from build123d import *

# Parameters (mm, degrees)
F0_W     = 10.859374
F0_H     = 12.747962
F1_DEPTH = 6.35


with BuildPart() as f1:
    # F0 (on Front) → F1 (new body)
    with BuildSketch(Plane.XZ):
        with Locations((-49.811488, 46.506466)):
            Rectangle(F0_W, F0_H)
        with BuildLine():
            ThreePointArc((-22.663044, 52.880447), (-33.522422, 50.119041), (-44.381801, 52.880447))
            Line((-44.381801, 52.880447), (-44.381801, 40.132485))
            ThreePointArc((-44.381801, 40.132485), (-33.58522, 42.779586), (-22.788638, 40.132485))
            Line((-22.788638, 40.132485), (-22.663044, 52.880447))
        make_face()
        Polygon((-12.275815, 52.880447), (-22.663044, 52.880447), (-22.788638, 40.132485), (-12.31831, 39.847307), align=None)
        Polygon((-12.31831, 39.847307), (-22.788638, 40.132485), (-22.788638, -13.626155), (-12.31831, -13.626155), align=None)
        with BuildLine():
            ThreePointArc((31.161692, 25.968079), (13.273611, 45.607102), (-12.275815, 52.880447))
            Line((-12.275815, 52.880447), (-12.31831, 39.847307))
            ThreePointArc((-12.31831, 39.847307), (10.459966, 36.160339), (31.161692, 25.968079))
        make_face()
        with BuildLine():
            Line((-12.31831, -13.626155), (-22.788638, -13.626155))
            ThreePointArc((-22.788638, -13.626155), (-27.217846, -15.308543), (-29.413201, -19.5072))
            Line((-29.413201, -19.5072), (-29.413201, -69.189601))
            ThreePointArc((-29.413201, -69.189601), (-28.519701, -72.668194), (-26.060402, -75.285599))
            Line((-26.060402, -75.285599), (-10.666025, -75.377978))
            ThreePointArc((-10.666025, -75.377978), (-8.094471, -72.573766), (-7.162803, -68.884797))
            Line((-7.162803, -68.884797), (-7.162803, -18.592801))
            ThreePointArc((-7.162803, -18.592801), (-8.738966, -15.069801), (-12.31831, -13.626155))
        make_face()
    extrude(amount=F1_DEPTH)


solid = f1.part
Geometry: final body of the model. Coordinates: model frame, mm. A direction names the side the tool comes from. Give positions to 0.01 mm unless a question says otherwise; leave off trailing zeros. Write each loop counter-clockwise with the first axis right and the second up, starting at its lowest first coordinate (ties: lowest second). Pieces come first, ordered by that corner, then holes. Notation, with made-up numbers: (4, 62.25) -> (46, 62.25) arc R26 ccw to (46, 94.25) -> close; hole circle Ø2 at (34.5, 36.5). An arc over 180 degrees is marked (long way). Answer in a Markdown table with one row per item.
(1) Ray query, line 1 along X through (y, z) = (-4.75, -57.5); line 2 along Z through (x, y) = (-48.5, -5); line 3 along X through (y, z) = (-4.25, -0.5). Return the intervals inside material, ascending. Write a range as [from, to].
Answers below:
| item | result |
|---|---|
| line 1 | [-29.41, -7.16] |
| line 2 | [40.13, 52.88] |
| line 3 | [-22.79, -12.32] |
(2) Section query B-B on y = -2.75. Return loops of the section in (x, z).
Answers below:
| item | result |
|---|---|
| outline | (-55.24, 40.13) -> (-44.38, 40.13) arc R23.34 cw to (-22.79, 40.13) -> (-22.79, -13.63) arc R6.67 ccw to (-29.41, -19.51) -> (-29.41, -69.19) arc R7.22 ccw to (-26.06, -75.29) -> (-10.67, -75.38) arc R7.77 ccw to (-7.16, -68.88) -> (-7.16, -18.59) arc R5.16 ccw to (-12.32, -13.63) -> (-12.32, 39.85) arc R77.97 cw to (31.16, 25.97) arc R48.51 ccw to (-12.28, 52.88) -> (-22.66, 52.88) arc R22.73 cw to (-44.38, 52.88) -> (-55.24, 52.88) -> close |
(3) Pin query (flat end, axial travel): pin 1 (1.9 mm diameter, centred on x = -48, y = -2.5, fed in from -Z); pin 2 (1.9 mm diameter, centred on y = -3.5, z = -33, fed in from +X); pin 3 (3 mm diameter, centred on x = 1.5, y = -5, fed in from +Z). Return the tip coordinate at first contact, or that it passes through.
Answers below:
| item | result |
|---|---|
| pin 1 | z = 40.13 |
| pin 2 | x = -7.16 |
| pin 3 | z = 51.3 |
(4) Set-up query: faces 1 (the flat face through (-50, -3, 40.132)), 2 (the flat face through (-7.163, -3, -44)), 3 (the flat face through (-12.318, -3, 13)), 4 (the cylindrical face through (-27.167, -3.131, -15.264)), 5 (the flat face through (-19, -6.35, -6)). Return all of +Z, -Z, +X, -X, +Y, -Y with unobstructed straight access to the full face (end or side cutting, diameter ignored); none if empty.
Answers below:
| item | result |
|---|---|
| face 1 | -Z, -X, +Y, -Y |
| face 2 | -Z, +X, +Y, -Y |
| face 3 | +Y, -Y |
| face 4 | -X, +Y, -Y |
| face 5 | +Z, -Z, +X, -X, -Y |
(5) Section query A-A on z = 36. Return loops of the section in (x, y), then the cut area to 3 significant figures.
Answers below:
| item | result |
|---|---|
| outline | (-22.79, -6.35) -> (-12.32, -6.35) -> (-12.32, 0) -> (-22.79, 0) -> close; (10.96, -6.35) -> (24.5, -6.35) -> (24.5, 0) -> (10.96, 0) -> close |
| area | 153 mm^2 |
(6) Draft query along Z for faces 6 (the flat face through (-55.241, -3, 46)), 7 (the flat face through (-22.789, -3, 14)), 8 (the cylindrical face through (13.59, -3.13, 45.41)). Return one class per face: +Z half, -Z half, draft (parallel to the pull), parting line (faces both ways), or undercut.
Answers below:
| item | result |
|---|---|
| face 6 | draft |
| face 7 | undercut |
| face 8 | +Z half |
(7) Section query C-C on x = -46. Return loops of the section in (y, z).
Answers below:
| item | result |
|---|---|
| outline | (-6.35, 40.13) -> (0, 40.13) -> (0, 52.88) -> (-6.35, 52.88) -> close |
(8) Section query D-D on z = -53.5. Return loops of the section in (x, y).
Answers below:
| item | result |
|---|---|
| outline | (-29.41, -6.35) -> (-7.16, -6.35) -> (-7.16, 0) -> (-29.41, 0) -> close |
